```python
from build123d import *

# Parameters (mm, degrees)
SKETCH1_R           = 1.6
BOSS_EXTRUDE1_DEPTH = 4.5
CUT_EXTRUDE1_DEPTH  = 10
FILLET1_R           = 1


with BuildPart() as part:
    # Sketch1 → Boss-Extrude1 (new body)
    with BuildSketch(Plane(origin=(0, 0, 0), x_dir=(1, 0, 0), z_dir=(0, 1, 0))):
        with BuildLine():
            Line((3.359522367, -0.523076923), (2.371427553, -6.869230769))
            ThreePointArc((2.371427553, -6.869230769), (1.561064725, -8.322930861), (0, -8.9))
            Line((0, -8.9), (-20, -8.9))
            ThreePointArc((-20, -8.9), (-22.4, -6.5), (-20, -4.1))
            Line((-20, -4.1), (-11.8, -4.1))
            Line((-11.8, -4.1), (-11.8, 1.4))
            Line((-11.8, 1.4), (-9.8, 1.4))
            Line((-9.8, 1.4), (-6.8, 0.4))
            Line((-6.8, 0.4), (-6.8, 0.3))
            ThreePointArc((-6.8, 0.3), (-7.063603897, -0.336396103), (-7.7, -0.6))
            Line((-7.7, -0.6), (-7.8, -0.6))
            Line((-7.8, -0.6), (-7.8, -4.1))
            Line((-7.8, -4.1), (-4.079334467, -4.1))
            Line((-4.079334467, -4.1), (-3.359522367, 0.523076923))
            ThreePointArc((-3.359522367, 0.523076923), (0.523076923, 3.359522367), (3.359522367, -0.523076923))
        make_face()
        with Locations(Location((0, 0, 0), (0, 0, 270))):
            Circle(SKETCH1_R, mode=Mode.SUBTRACT)
    extrude(amount=BOSS_EXTRUDE1_DEPTH)

    # Sketch2 → Cut-Extrude1 (cut)
    with BuildSketch(Plane(origin=(0, 4.5, 0), x_dir=(1, 0, 0), z_dir=(0, 1, 0))):
        Polygon((-3.359522367, 0.523076923), (-3.359522367, -4.1), (-4.079334467, -4.1), align=None)
    extrude(amount=-CUT_EXTRUDE1_DEPTH, mode=Mode.SUBTRACT)

    # Fillet1
    fillet1_edges = [part.edges().sort_by_distance(p)[0] for p in [
        (-3.359522367, 2.25, 4.1),
    ]]
    fillet(fillet1_edges, radius=FILLET1_R)


solid = part.part
```
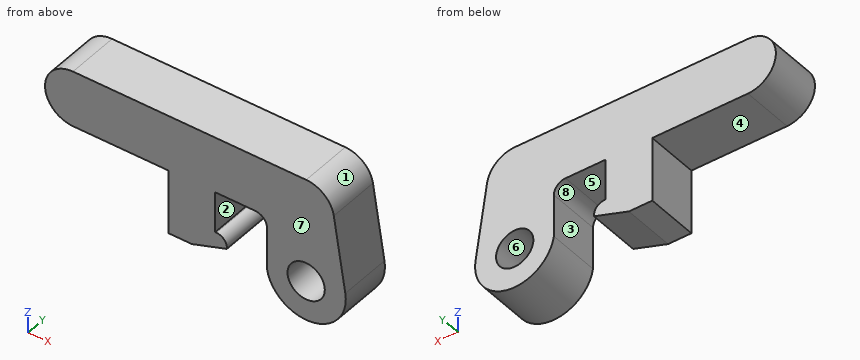
Verification items for the finished model (mm, model axes). Face numbers are marked on the shaded views. A direction names the side the tool comes from. Coordinates: 2 decimals unless noted, no trailing zeros. Order: outer loops, then holes, each group sorted by start corner. A loop starts at its lowest first (then second) coordinate and runs counter-clockwise, first axis right, second up. Notation, with made-up numbers: (81, 54) -> (134, 54) arc R22 cw to (134, 71) -> close; hole circle Ø11 at (-0.75, -19). An arc over 180 degrees is marked (long way). Answer as CSV lines item,"result". Start each with the question number.
1) Release check for a two-part mould opening along Z. For the marked faces 5, 6, 7 and 8 record: released by +Z, released by -Z, zero draft, split by the parting line, or undercut.
2) Cross-section at D-D, the plane z = 6.5. Record the boundary of the cut face in (x, y), then the cut area to 3 significant figures.
3) Cross-section at A-A, the plane z = 0. Record the boundary of the cut face in (x, y).
4) Set-up check for the marked faces 1, 2, 3 and 4: record each of +Z, -Z, +X, -X, +Y, -Y from which the full face is reachable in a straight line by a thin tool's end or side.
5) Material ranges on L1, parallel to X at y = 1.2, z = 0; L2, parallel to Z at x = -10.5, y = 1.1; L3, parallel to Z at x = -15, y = 0.5, recorded low to high. Write a range as [from, to].
6) Cross-section at C-C, the plane x = -19.5. Record the boundary of the cut face in (y, z), then the cut area to 3 significant figures.
7) Gauge pin test, flat ends, axial feed: pin 1 Ø2 at (x, y) = (-14, 3.5) entering from -Z; pin 2 Ø1 at (x, z) = (-4.5, 4) entering from +Y; pin 3 Ø1 at (y, z) = (1, 2) entering from +X; pin 4 Ø1.6 at (x, y) = (-10.5, 2.5) entering from -Z. Record the tip position at first contact, or that the pin passes through.
8) Cross-section at B-B, the plane y = 4.15. Record the boundary of the cut face in (x, z).
Conclusion:
1,face 5,"undercut"
1,face 6,"undercut"
1,face 7,"zero draft"
1,face 8,"released by -Z"
2,outline,"(-22.4, 0) -> (2.43, 0) -> (2.43, 4.5) -> (-22.4, 4.5) -> close"
2,area,"112 mm²"
3,outline,"(-11.8, 0) -> (-6.85, 0) -> (-6.85, 4.5) -> (-11.8, 4.5) -> close; (-3.36, 0) -> (-1.6, 0) -> (-1.6, 4.5) -> (-3.36, 4.5) -> close; (1.6, 0) -> (3.4, 0) -> (3.4, 4.5) -> (1.6, 4.5) -> close"
4,face 1,"+Z, +X, +Y, -Y"
4,face 2,"+Y, -Y"
4,face 3,"-Z, +Y, -Y"
4,face 4,"-Z, -X, +Y, -Y"
5,L1,"x = [-11.8, -6.85], [-3.36, -1.6], [1.6, 3.4]"
5,L2,"z = [-1.4, 8.9]"
5,L3,"z = [4.1, 8.9]"
6,outline,"(0, 4.1) -> (4.5, 4.1) -> (4.5, 8.9) -> (0, 8.9) -> close"
6,area,"21.6 mm²"
7,pin 1,"stops at z = 4.1"
7,pin 2,"stops at y = 4.5"
7,pin 3,"stops at x = 3.21"
7,pin 4,"stops at z = -1.4"
8,outline,"(-20, 4.1) -> (-11.8, 4.1) -> (-11.8, -1.4) -> (-9.8, -1.4) -> (-6.8, -0.4) -> (-6.8, -0.3) arc R0.9 ccw to (-7.7, 0.6) -> (-7.8, 0.6) -> (-7.8, 4.1) -> (-4.36, 4.1) arc R1 cw to (-3.36, 3.1) -> (-3.36, -0.52) arc R3.4 ccw to (3.36, 0.52) -> (2.37, 6.87) arc R2.4 ccw to (0, 8.9) -> (-20, 8.9) arc R2.4 ccw to start; hole circle Ø3.2 at (0, 0)"
